Input: part model. Units: mm. Frame: model coordinates. Face numbers are marked on the shaded views. A direction names the side the tool comes from. Coordinates: 2 decimals unless noted, no trailing zeros. Order: outer loops, then holes, each group sorted by start corner. A loop starts at its lowest first (then second) coordinate and runs counter-clockwise, first axis right, second up.
Autodesk Inventor part; units mm, degrees
ref_plane "YZ Plane" through (0, 0, 0) normal (1, 0, 0) x (0, 1, 0)
ref_plane "XZ Plane" through (0, 0, 0) normal (0, 1, 0) x (-1, 0, 0)
ref_plane "XY Plane" through (0, 0, 0) normal (0, 0, 1) x (1, 0, 0)
sketch "Sketch1" plane through (0, 0, 0) normal (0, 1, 0) x (-1, 0, 0)
  line L0 (92.3312, 46.4889) -> (54.1312, 46.4889)
  line L1 (54.1312, 46.4889) -> (54.1312, 103.4889)
  line L2 (54.1312, 103.4889) -> (92.3312, 103.4889)
  line L3 (92.3312, 103.4889) -> (92.3312, 46.4889)
  circle A0 centre (89.1312, 49.5389) radius 1.6
  circle A1 centre (57.3312, 49.5389) radius 1.6
  circle A2 centre (89.1312, 100.4389) radius 1.6
  circle A3 centre (57.3312, 100.4389) radius 1.6
  point P0 (0, 0)
  dimension "d0" = 57
  dimension "d1" = 38.2
  dimension "d2" = 3.2
  dimension "d3" = 3.2
  dimension "d4" = 3.05
  dimension "d11" = 3.05
  dimension "d12" = 3.2
  dimension "d13" = 3.05
  dimension "d14" = 3.05
  dimension "d15" = 3.2
  dimension "d16" = 3.2
extrude "Extrusion1" add sketch "Sketch1" along normal blind 1.6
sketch "Sketch2" plane through (0, 1.6, 0) normal (0, 1, 0) x (1, 0, 0)
  line L0 (-81.0812, -52.6889) -> (-65.3812, -52.6889)
  line L1 (-65.3812, -52.6889) -> (-65.3812, -65.0889)
  line L2 (-65.3812, -65.0889) -> (-81.0812, -65.0889)
  line L3 (-81.0812, -65.0889) -> (-81.0812, -52.6889)
  line L4 (-54.1312, -46.4889) -> (-92.3312, -46.4889)
  line L5 (-92.3312, -46.4889) -> (-92.3312, -103.4889) construction
  line L6 (-54.1312, -46.4889) -> (-92.3312, -103.4889) construction
  line L7 (-92.3312, -103.4889) -> (-54.1312, -103.4889) construction
  line L8 (-92.3312, -46.4889) -> (-54.1312, -103.4889) construction
  line L9 (-73.2312, -103.4889) -> (-73.2312, -46.4889) construction
  point P0 (0, 0)
  point P1 (-73.2312, -52.6889)
  dimension "d19" = 6.2
  dimension "d20" = 15.7
  dimension "d21" = 12.4
extrude "Extrusion2" add sketch "Sketch2" along normal blind 21.2
sketch "Sketch3" plane through (0, 1.6, 0) normal (0, 1, 0) x (1, 0, 0)
  line L0 (-81.0812, -65.0889) -> (-65.3812, -65.0889)
  line L1 (-84.2537, -65.0889) -> (-62.2087, -65.0889)
  line L2 (-62.2087, -65.0889) -> (-62.2087, -96.5889)
  line L3 (-62.2087, -96.5889) -> (-84.2537, -96.5889)
  line L4 (-84.2537, -96.5889) -> (-84.2537, -65.0889)
  line L5 (-92.3312, -103.4889) -> (-54.1312, -103.4889)
  line L6 (-54.1312, -103.4889) -> (-54.1312, -46.4889) construction
  line L7 (-54.1312, -103.4889) -> (-92.3312, -46.4889) construction
  line L8 (-92.3312, -103.4889) -> (-54.1312, -46.4889) construction
  line L9 (-73.2312, -61.8477) -> (-73.2312, -121.9284) construction
  point P0 (0, 0)
  dimension "d24" = 6.9
extrude "Extrusion3" add sketch "Sketch3" along normal blind 14
properties part number "NAS_Splitter_PCB"
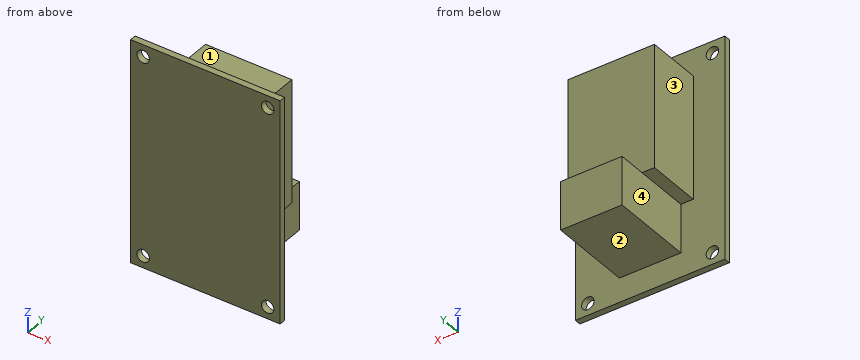
Item 1: Cut plane C-C on z = 74. Return loops of the section in (x, y), then the cut area to 3 significant figures.
Response values:
outline: (-92.33, 0) - (-54.13, 0) - (-54.13, 1.6) - (-62.21, 1.6) - (-62.21, 15.6) - (-84.25, 15.6) - (-84.25, 1.6) - (-92.33, 1.6) - close
area: 370 mm2
Item 2: Cut plane A-A on y = 5.5. Return loops of the section in (x, z), then the cut area to 3 significant figures.
Response values:
outline: (-84.25, 65.09) - (-81.08, 65.09) - (-81.08, 52.69) - (-65.38, 52.69) - (-65.38, 65.09) - (-62.21, 65.09) - (-62.21, 96.59) - (-84.25, 96.59) - close
area: 889 mm2
Item 3: Cut plane D-D on x = -71. Return loops of the section in (y, z), then the cut area to 3 significant figures.
Response values:
outline: (0, 46.49) - (1.6, 46.49) - (1.6, 52.69) - (22.8, 52.69) - (22.8, 65.09) - (15.6, 65.09) - (15.6, 96.59) - (1.6, 96.59) - (1.6, 103.49) - (0, 103.49) - close
area: 795 mm2
Item 4: Pin query (flat end, axial travel): pin 1 Ø4 at (y, z) = (5, 73) entering from +X; pin 2 Ø1.5 at (y, z) = (6, 74.5) entering from -X; pin 3 Ø10 at (x, y) = (-67.5, 10) entering from -Z. Return the tip coordinate at first contact, or that it passes through.
Response values:
pin 1: stops at x = -62.21
pin 2: stops at x = -84.25
pin 3: stops at z = 52.69
Item 5: Cut plane B-B on x = -56.5. Return loops of the section in (y, z), then the cut area to 4 significant figures.
Response values:
outline: (0, 46.49) - (1.6, 46.49) - (1.6, 48.17) - (0, 48.17) - close; (0, 50.91) - (1.6, 50.91) - (1.6, 99.07) - (0, 99.07) - close; (0, 101.81) - (1.6, 101.81) - (1.6, 103.49) - (0, 103.49) - close
area: 82.45 mm2
Item 6: Access query for the marked faces 1, 2, 3 and 4. Directions: +Z, -Z, +X, -X, +Y, -Y. A direction counts if a zero-diameter tool reaches every point of the face in a straight line with its end or side. Return the directions, or none.
Response values:
face 1: +Z, +X, -X, +Y
face 2: -Z, +X, -X, +Y
face 3: +Z, -Z, -X, +Y
face 4: -Z, -X, +Y
Item 7: Ray query, probe 1 along Z at (x, y) = (-65.5, 13); probe 2 along Y at (x, z) = (-89, 75.5); probe 3 along Z at (x, y) = (-77.5, 17). Return the intervals inside material, ascending.
Response values:
probe 1: z = 52.69 to 96.59
probe 2: y = 0 to 1.6
probe 3: z = 52.69 to 65.09
